Job drawing, mm, ordinate dimensions from the low corner. One solid piece. Give positions to 0.01 mm unless a question says otherwise; leave off trailing zeros. Loops run counter-clockwise (first coordinate to the right, second up) from the corner with the lowest first, then second, coordinate; pieces in that order, holes last. Notation, with made-up numbers: (70, 34) - (91, 34) arc R26 cw to (91, 72) - close; hole circle Ø4 at (1.25, -37.75). An arc over 180 degrees is marked (long way). Use a Markdown table: item, result.
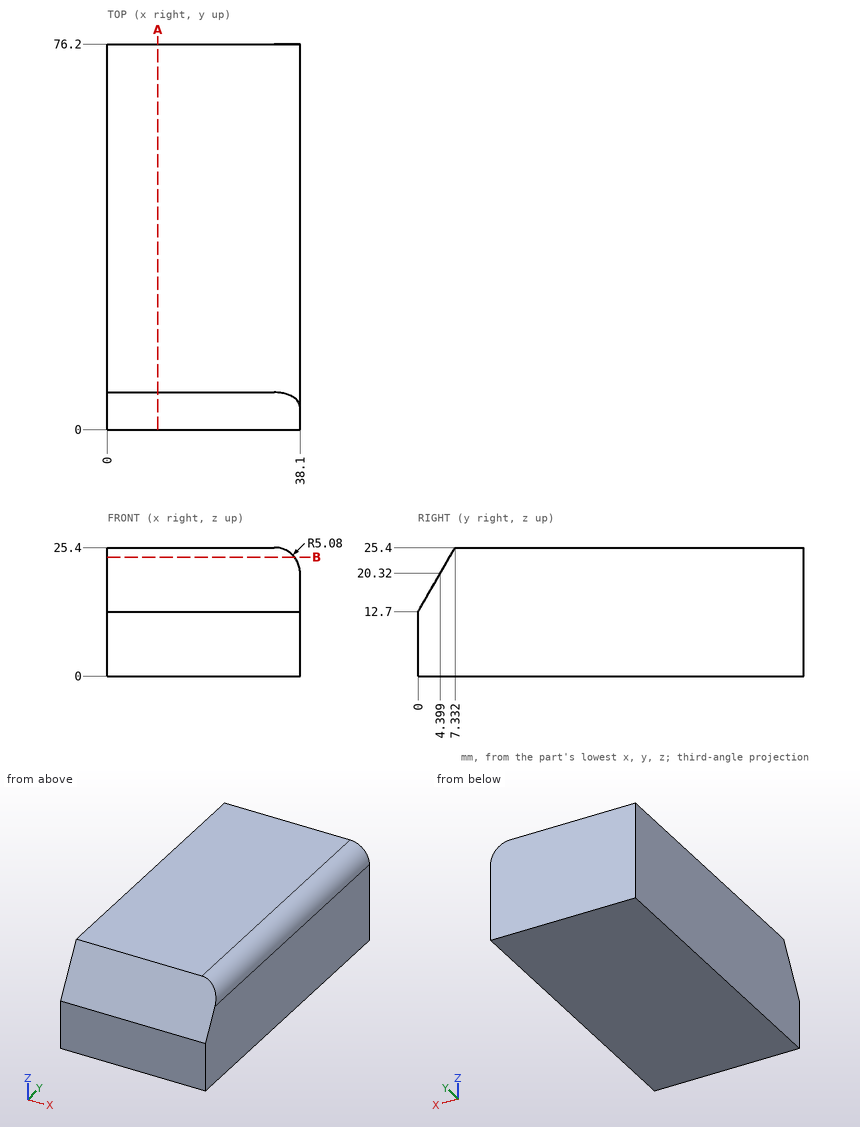
(1) Drill centre lines: probe 1 along X at (y, z) = (70.5, 20.5); probe 2 along Y at (x, z) = (21.5, 22.5); probe 3 along Y at (x, z) = (8.5, 20) (1 decimal). Where is each one in solid material? Low to high. Write a range as [from, to].
Computed:
| item | result |
|---|---|
| probe 1 | [0, 38.1] |
| probe 2 | [5.66, 76.2] |
| probe 3 | [4.2, 76.2] |
(2) Slice it at B-B, the plane z = 23.5. Write the cut outline in (x, y) (1 decimal).
Computed:
| item | result |
|---|---|
| outline | (0, 6.2) - (37, 6.2) - (37, 76.2) - (0, 76.2) - close |
(3) Pin check, flat tip, straight feed: P1, Ø4, axis at x = 25, y = 54.5, coming from the -Z side. Stop position of the tip, or through.
Computed:
| item | result |
|---|---|
| P1 | z = 0 |
(4) Slice it at A-A, the plane x = 10. Write the cut outline in (y, z), plus the area to 3 significant figures.
Computed:
| item | result |
|---|---|
| outline | (0, 0) - (76.2, 0) - (76.2, 25.4) - (7.33, 25.4) - (0, 12.7) - close |
| area | 1,890 mm² |
